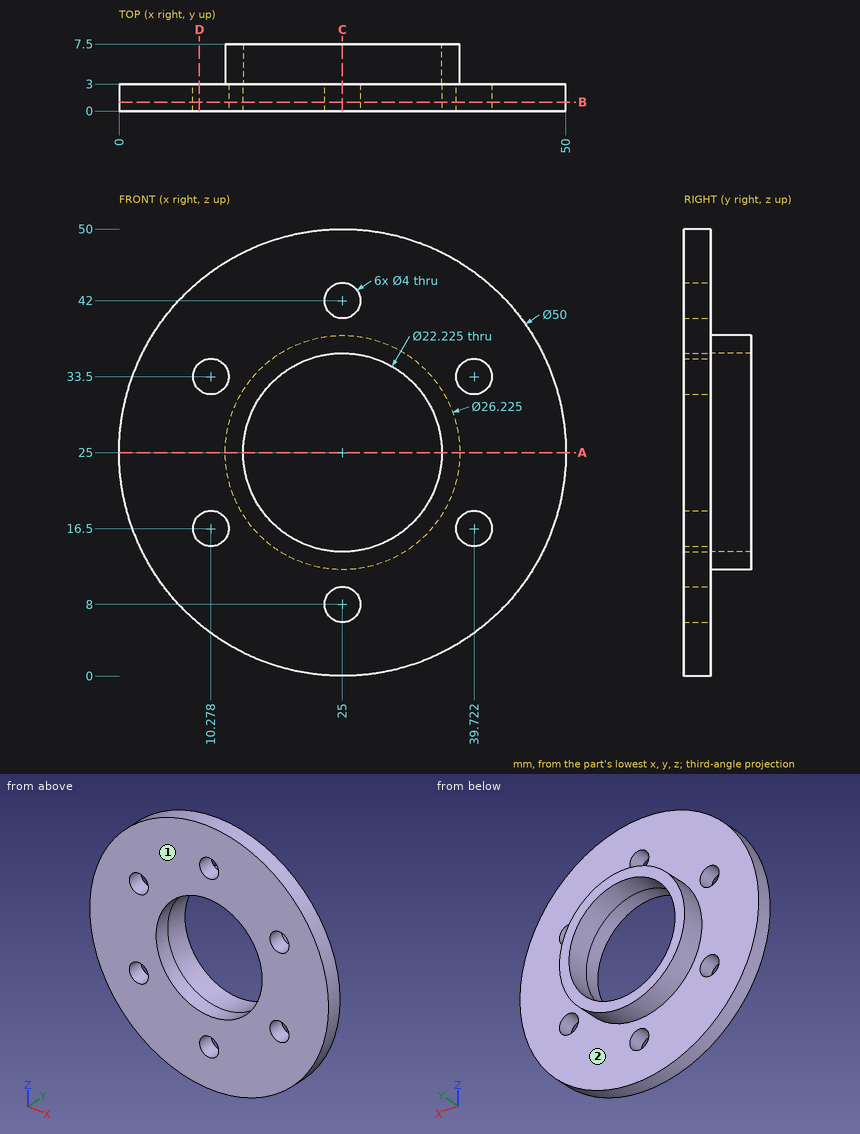
Verification items for this drawing (mm, ordinates from the low corner). A direction names the side the tool comes from. Give positions to 0.01 mm unless a question says otherwise; leave off trailing zeros. Loops run counter-clockwise (first coordinate to the right, second up) from the corner with the lowest first, then second, coordinate; pieces in that order, holes last.
1. Go/stop test with flat-tipped pins: P1, Ø2, axis at y = 6, z = 10, coming from the +X side; P2, Ø1, axis at x = 18.5, y = 5, coming from the +Z side; P3, Ø6.5, axis at x = 25, z = 8, coming from the +Y side; P4, Ø1.5, axis at y = 5.5, z = 15, coming from the +X side (1 decimal). Record where each tip stops, or that it passes through.
Derived:
P1: passes through
P2: stops at z = 36.66
P3: stops at y = 3
P4: stops at x = 34.3
2. Cross-section at A-A on z = 25. Record the cut outline in (x, y), and give its area (3 significant figures).
Derived:
outline: (0, 0) - (13.89, 0) - (13.89, 7.5) - (11.89, 7.5) - (11.89, 3) - (0, 3) - close; (36.11, 0) - (50, 0) - (50, 3) - (38.11, 3) - (38.11, 7.5) - (36.11, 7.5) - close
area: 101 mm2
3. Tool access check on the marked faces 1 and 2. Record the directions out of +Z, -Z, +X, -X, +Y, -Y that give a thin tool (end or side, any length) a straight path to the whole face; none if there is none.
Derived:
face 1: +Z, -Z, +X, -X, -Y
face 2: +Y
4. Material ranges on probe 1 along Z at (x, y) = (25, 2.25); probe 2 along X at (y, z) = (2.5, 33) (1 decimal); probe 3 along Y at (x, z) = (39.5, 12), recorded low to high.
Derived:
probe 1: z = 0 to 6, 10 to 13.89, 36.11 to 40, 44 to 50
probe 2: x = 1.3 to 8.3, 12.2 to 17.3, 32.7 to 37.8, 41.7 to 48.7
probe 3: y = 0 to 3
5. Cross-section at B-B on y = 1. Record the cut outline in (x, z) (1 decimal), and give its area (3 significant figures).
Derived:
outline: circle Ø50 at (25, 25); hole circle Ø4 at (10.3, 16.5); hole circle Ø4 at (10.3, 33.5); hole circle Ø22.2 at (25, 25); hole circle Ø4 at (25, 8); hole circle Ø4 at (25, 42); hole circle Ø4 at (39.7, 16.5); hole circle Ø4 at (39.7, 33.5)
area: 1,500 mm2
6. Cross-section at D-D on x = 9. Record the cut outline in (y, z).
Derived:
outline: (0, 5.79) - (3, 5.79) - (3, 14.96) - (0, 14.96) - close; (0, 18.04) - (3, 18.04) - (3, 31.96) - (0, 31.96) - close; (0, 35.04) - (3, 35.04) - (3, 44.21) - (0, 44.21) - close
7. Cross-section at C-C on x = 25. Record the cut outline in (y, z).
Derived:
outline: (0, 0) - (3, 0) - (3, 6) - (0, 6) - close; (0, 10) - (3, 10) - (3, 11.89) - (7.5, 11.89) - (7.5, 13.89) - (0, 13.89) - close; (0, 36.11) - (7.5, 36.11) - (7.5, 38.11) - (3, 38.11) - (3, 40) - (0, 40) - close; (0, 44) - (3, 44) - (3, 50) - (0, 50) - close
